Source: CAD feature listing. Evaluate the final solid. Frame: model axes, mm. A direction names the side the tool comes from. Give positions to 0.01 mm unless a question says otherwise; leave off trailing zeros. Order: outer loops, then holes, each group sorted by start corner. A loop starts at its lowest first (then second) coordinate and runs counter-clockwise, first axis right, second up.
from build123d import *

# Parameters (mm, degrees)
BOSS_EXTRUDE1_DEPTH = 3


with BuildPart() as part:
    # Sketch1 → Boss-Extrude1 (new body)
    with BuildSketch(Plane.XY):
        Polygon((219, 51), (219, 48), (216, 48), (216, 45), (219, 45), (219, 42), (216, 42), (216, 39), (219, 39), (219, 36), (216, 36), (216, 33), (219, 33), (219, 30), (216, 30), (216, 27), (219, 27), (219, 24), (216, 24), (216, 21), (219, 21), (219, 18), (216, 18), (216, 15), (219, 15), (219, 12), (216, 12), (216, 9), (219, 9), (219, 6), (222, 6), (222, 3), (225, 3), (225, 6), (228, 6), (228, 3), (231, 3), (231, 6), (234, 6), (234, 3), (237, 3), (237, 6), (240, 6), (240, 3), (243, 3), (243, 6), (246, 6), (246, 3), (249, 3), (249, 6), (252, 6), (252, 3), (255, 3), (255, 6), (258, 6), (258, 3), (261, 3), (261, 6), (264, 6), (264, 3), (267, 3), (267, 6), (270, 6), (270, 3), (273, 3), (273, 6), (276, 6), (276, 3), (279, 3), (279, 6), (282, 6), (282, 3), (285, 3), (285, 6), (288, 6), (288, 9), (291, 9), (291, 12), (288, 12), (288, 15), (291, 15), (291, 18), (288, 18), (288, 21), (291, 21), (291, 24), (288, 24), (288, 27), (291, 27), (291, 30), (288, 30), (288, 33), (291, 33), (291, 36), (288, 36), (288, 39), (291, 39), (291, 42), (288, 42), (288, 45), (291, 45), (291, 48), (288, 48), (288, 51), (291, 51), (291, 54), (288, 54), (288, 57), (291, 57), (291, 60), (288, 60), (288, 63), (291, 63), (291, 66), (288, 66), (288, 69), (291, 69), (291, 72), (288, 72), (288, 75), (285, 75), (285, 78), (282, 78), (282, 75), (279, 75), (279, 78), (276, 78), (276, 75), (273, 75), (273, 78), (270, 78), (270, 75), (267, 75), (267, 78), (264, 78), (264, 75), (261, 75), (261, 78), (258, 78), (258, 75), (255, 75), (255, 78), (252, 78), (252, 75), (249, 75), (249, 78), (246, 78), (246, 75), (243, 75), (243, 78), (240, 78), (240, 75), (237, 75), (237, 78), (234, 78), (234, 75), (231, 75), (231, 78), (228, 78), (228, 75), (225, 75), (225, 78), (222, 78), (222, 75), (219, 75), (219, 72), (216, 72), (216, 69), (219, 69), (219, 66), (216, 66), (216, 63), (219, 63), (219, 60), (216, 60), (216, 57), (219, 57), (219, 54), (216, 54), (216, 51), align=None)
    extrude(amount=BOSS_EXTRUDE1_DEPTH)


solid = part.part
(1) Section A-A, the plane y = 62. Return loops of the section in (x, z).
(2) Section B-B, the plane x = 256.5. Return loops of the section in (y, z).
(3) Pin query (flat end, axial travel): pin 1 Ø0.9 at (y, z) = (14, 2) entering from -X; pin 2 Ø0.9 at (y, z) = (25, 1) entering from +X; pin 3 Ø0.9 at (y, z) = (4, 2) entering from -X. Return the tip coordinate at first contact, or that it passes through.
(4) Access query for faces 5 (the flat face through (216, 59, 1)), 6 (the flat face through (217, 27, 1)), 7 (the flat face through (244, 6, 1)), 8 (the flat face through (285, 76, 1)), 9 (the flat face through (288, 49, 1)). Directions: +Z, -Z, +X, -X, +Y, -Y. A direction counts if a zero-diameter tool reaches every point of the face in a straight line with its end or side. Return the directions, or none.
(5) Line query: line 1 along X through (y, z) = (55.5, 0.4); line 2 along Y through (x, z) = (244, 0.4). Output: solid intervals per line, ascending.
(6) Draft query along Y for faces 1 (the flat face through (229, 3, 1)), 2 (the flat face through (289, 15, 1)), 3 (the flat face through (291, 28, 1)), 4 (the flat face through (278, 78, 1)). Return one class per face: +Y half, -Y half, draft (parallel to the pull), parting line (faces both ways), or undercut.
Checks:
1. outline: (219, 0) - (288, 0) - (288, 3) - (219, 3) - close
2. outline: (6, 0) - (75, 0) - (75, 3) - (6, 3) - close
3. pin 1: stops at x = 219
3. pin 2: stops at x = 288
3. pin 3: stops at x = 222
4. face 5: +Z, -Z, -X, +Y, -Y
4. face 6: +Z, -Z, -X
4. face 7: +Z, -Z, -Y
4. face 8: +Z, -Z, +X, +Y
4. face 9: +Z, -Z, +X
5. line 1: x = 219 to 288
5. line 2: y = 6 to 75
6. face 1: -Y half
6. face 2: undercut
6. face 3: draft
6. face 4: +Y half
